Input: dimensioned drawing with shaded views. Units: mm. Origin: part minimum x, y, z. A direction names the side the tool comes from. Give positions to 0.01 mm unless a question says otherwise; leave off trailing zeros. Loops run counter-clockwise (first coordinate to the right, second up) from the corner with the lowest first, then second, coordinate; pieces in that order, holes last. Notation, with made-up numbers: (-17.5, 83) -> (8.5, 83) arc R32 cw to (8.5, 117) -> close; hole circle Ø4 at (76.25, 31.25). An arc over 180 degrees is marked (long way). Answer as a JSON object with one key per item and string values.
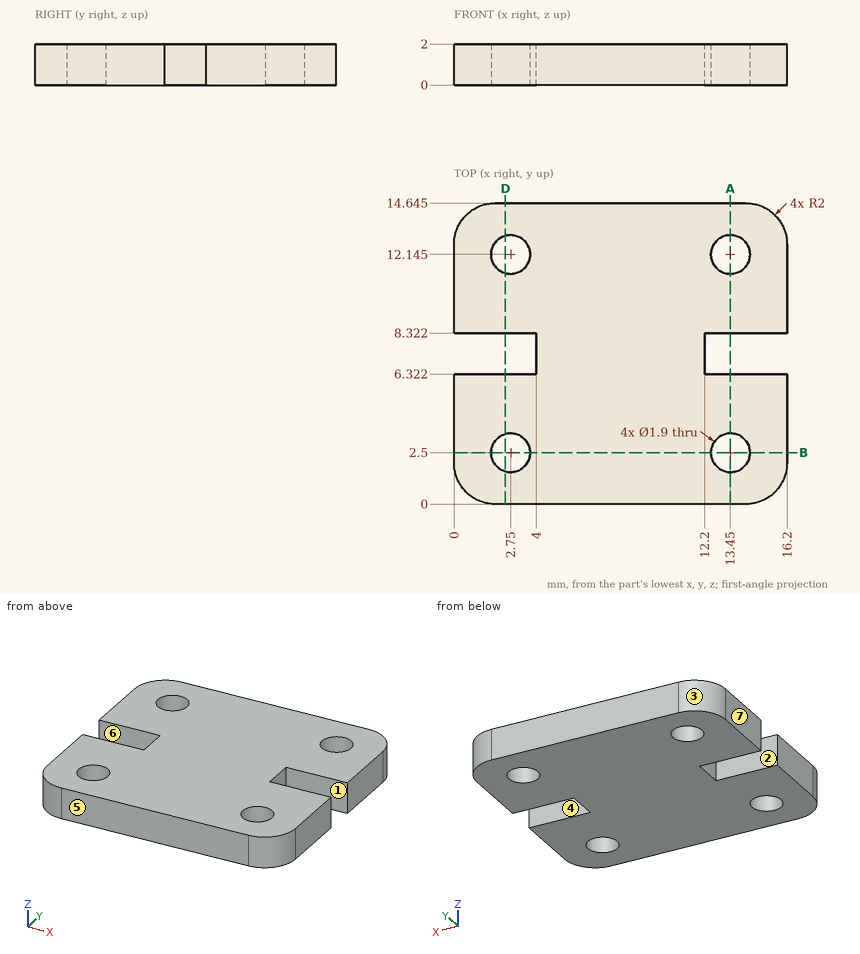
Q1. Access query for the marked faces 1, 2 and 3. Directions: +Z, -Z, +X, -X, +Y, -Y. A direction counts if a zero-diameter tool reaches every point of the face in a straight line with its end or side. Return the directions, or none.
Evaluation:
{"face 1": "+Z, -Z, +X", "face 2": "+Z, -Z, -X", "face 3": "+Z, -Z, -X, +Y"}
Q2. Ray query, line 1 along X through (y, z) = (2.5, 1.6); line 2 along X through (y, z) = (12.75, 1.75) (1 decimal); line 3 along X through (y, z) = (8.25, 1.85). Return the intervals inside material, ascending.
Evaluation:
{"line 1": "x = 0 to 1.8, 3.7 to 12.5, 14.4 to 16.2", "line 2": "x = 0 to 2, 3.5 to 12.7, 14.2 to 16.2", "line 3": "x = 4 to 12.2"}
Q3. Section B-B, the plane y = 2.5. Return the cut outline in (x, z), then the cut area to 3 significant figures.
Evaluation:
{"outline": "(0, 0) -> (1.8, 0) -> (1.8, 2) -> (0, 2) -> close; (3.7, 0) -> (12.5, 0) -> (12.5, 2) -> (3.7, 2) -> close; (14.4, 0) -> (16.2, 0) -> (16.2, 2) -> (14.4, 2) -> close", "area": "24.8 mm2"}
Q4. Section D-D, the plane x = 2.5. Return the cut outline in (y, z) (1 decimal).
Evaluation:
{"outline": "(0, 0) -> (1.6, 0) -> (1.6, 2) -> (0, 2) -> close; (3.4, 0) -> (6.3, 0) -> (6.3, 2) -> (3.4, 2) -> close; (8.3, 0) -> (11.2, 0) -> (11.2, 2) -> (8.3, 2) -> close; (13.1, 0) -> (14.6, 0) -> (14.6, 2) -> (13.1, 2) -> close"}
Q5. Draft query along Y for the marked faces 4, 5, 6 and 7. Return one class per face: +Y half, -Y half, draft (parallel to the pull), parting line (faces both ways), or undercut.
Evaluation:
{"face 4": "undercut", "face 5": "-Y half", "face 6": "undercut", "face 7": "draft"}
Q6. Section A-A, the plane x = 13.45. Give the number of separate pieces and of enclosed holes in the cut face, then the cut area to 3 significant figures.
Evaluation:
{"separate pieces": "4", "enclosed holes": "0", "area": "17.7 mm2"}
